Here's how the part is built. I have some questions about the finished solid (model axes, mm). Round coordinates to 2 decimals unless told otherwise and drop trailing zeros. Write each loop counter-clockwise with the first axis right and the second up, starting at its lowest first coordinate (ties: lowest second). Pieces come first, ordered by that corner, then holes. Notation, with made-up numbers: M 0.5,43 L 26.5,43 A28 cw 26.5,69 Z; hole C 43.5,20.25 d1. An arc over 180 degrees is marked long. Use one line per item in the form item = value. Start each with the question number.
Q1. I want a section at B-B on y = 114.3. List the corners of the cut face in (x, z) for me, and give its area (3 significant figures).
Q2. I want a section at D-D on z = 1. State how many separate pieces and enclosed holes the cut face has, and give its area (3 significant figures).
Q3. I want a section at C-C on y = -101.6. List the corners of the cut face in (x, z) for me (3 decimals).
Q4. I'm going to push a flat-ended pin straight in: pin 1 Ø17 at (x, y) = (-165.1, 114.3) entering from +Z. Where does the tip first touch, or does it pass through?
Q5. I need wall thicknesses on line 1 along X through (y, z) = (-42, 5.5); line 2 along Y through (x, z) = (-165.1, 2); line 3 along X through (y, z) = (-48, 5.25). Which ranges of each line are inside material? Lowest first, please. Write a range as from..to.
Q6. We'd pull the mould along X, two halves only. Please class faces 1 (the face through (-4, 2, 6.35)), 2 (the face through (-228.1, 108.83, 3.13)), 3 (the face through (-113.8, 108.83, 3.13)): +X half, -X half, draft (parallel to the pull), parting line (faces both ways), or undercut.
Q7. I want a section at A-A on x = 0. List the corners of the cut face in (y, z) for me (3 decimals), and give its area (3 significant figures).
```python
from build123d import *

# Parameters (mm, degrees)
SKETCH_W   = 558.8
SKETCH_H   = 304.8
SKETCH_R   = 14.2875
SKETCH_R_2 = 15.875
SKETCH_R_3 = 12.7
PAD_DEPTH  = 6.35


with BuildPart() as part:
    # Sketch → Pad (new body)
    with BuildSketch(Plane.XY):
        Rectangle(SKETCH_W, SKETCH_H)
        with Locations((-241.3, 114.3)):
            Circle(SKETCH_R, mode=Mode.SUBTRACT)
        with Locations((-203.2, 114.3)):
            Circle(SKETCH_R, mode=Mode.SUBTRACT)
        with Locations((-127, 114.3)):
            Circle(SKETCH_R, mode=Mode.SUBTRACT)
        with Locations((-165.1, 114.3)):
            Circle(SKETCH_R, mode=Mode.SUBTRACT)
        with Locations((241.3, 114.3)):
            Circle(SKETCH_R, mode=Mode.SUBTRACT)
        with Locations((0, -101.6)):
            Circle(SKETCH_R_2, mode=Mode.SUBTRACT)
        with Locations((-215.9, -12.7)):
            Circle(SKETCH_R_3, mode=Mode.SUBTRACT)
        with Locations((69.85, -12.7)):
            Circle(SKETCH_R_3, mode=Mode.SUBTRACT)
        with Locations((-139.7, -12.7)):
            Circle(SKETCH_R, mode=Mode.SUBTRACT)
        with Locations((-102.485024, -20.864286)):
            Circle(SKETCH_R, mode=Mode.SUBTRACT)
        with Locations((-72.105452, -43.85758)):
            Circle(SKETCH_R, mode=Mode.SUBTRACT)
        with Locations((146.05, -43.85758)):
            Circle(SKETCH_R, mode=Mode.SUBTRACT)
        with Locations((176.429572, -20.864286)):
            Circle(SKETCH_R, mode=Mode.SUBTRACT)
        with Locations((213.644548, -12.7)):
            Circle(SKETCH_R, mode=Mode.SUBTRACT)
    extrude(amount=PAD_DEPTH)


solid = part.part
```
Reported:
q1.outline = M -279.4,0 L -255.59,0 L -255.59,6.35 L -279.4,6.35 Z; M -227.01,0 L -217.49,0 L -217.49,6.35 L -227.01,6.35 Z; M -188.91,0 L -179.39,0 L -179.39,6.35 L -188.91,6.35 Z; M -150.81,0 L -141.29,0 L -141.29,6.35 L -150.81,6.35 Z; M -112.71,0 L 227.01,0 L 227.01,6.35 L -112.71,6.35 Z; M 255.59,0 L 279.4,0 L 279.4,6.35 L 255.59,6.35 Z
q1.area = 2,640 mm^2
q2.separate_pieces = 1
q2.enclosed_holes = 14
q2.area = 161,000 mm^2
q3.outline = M -279.4,0 L -15.875,0 L -15.875,6.35 L -279.4,6.35 Z; M 15.875,0 L 279.4,0 L 279.4,6.35 L 15.875,6.35 Z
q4.pin_1 = through
q5.line_1 = -279.4..-86.27, -57.94..131.88, 160.22..279.4
q5.line_2 = -152.4..100.01, 128.59..152.4
q5.line_3 = -279.4..-85.78, -58.43..132.38, 159.72..279.4
q6.face_1 = draft
q6.face_2 = undercut
q6.face_3 = undercut
q7.outline = M -152.4,0 L -117.475,0 L -117.475,6.35 L -152.4,6.35 Z; M -85.725,0 L 152.4,0 L 152.4,6.35 L -85.725,6.35 Z
q7.area = 1,730 mm^2
